Geometry check sheet. Reference: the model listing, model coordinates, mm. Face numbers are marked on the shaded views. A direction names the side the tool comes from. Give positions to 0.01 mm unless a question says otherwise; leave off trailing zeros. Order: outer loops, then holes, each group sorted by start corner. A loop starts at its lowest first (then second) coordinate and runs counter-clockwise, first axis right, second up. Notation, with made-up numbers: M -8,84.5 L -1,84.5 A20 cw -1,104.5 Z; hole C -16.5,51 d4. An arc over 180 degrees is marked long. Put each result on its own line as item: value. Start each with the question number.
Q1. Section check B-B on y = -164. Record the cut outline in (x, z), then the cut area to 3 significant figures.
Q2. Section check D-D on z = -3.25. Record the cut outline in (x, y), then the cut area to 3 significant figures.
Q3. Section check A-A on x = 0.75. Record the cut outline in (y, z), then the cut area to 3 significant figures.
Q4. Go/stop test with a flat-tipped pin: pin 1 (13.5 mm diameter, centred on y = -254, z = 0, fed in from +X). Record where the tip stops, or that it passes through.
Q5. Section check C-C on y = -54. Record the cut outline in (x, z).
Q6. Material ranges on L1, parallel to Y at x = 13.9, z = 0; L2, parallel to Z at x = 3.5, y = -181, recorded low to high.
Q7. Access from +Z, -Z, +X, -X, +Y, -Y to the whole of each face (thin tool, end or side, straight path). Record for the marked faces 1 and 2.
Q8. Mould release check, pull along Z, two halves, no side actions. Record for the marked faces 3, 4 and 5: +Z half, -Z half, draft (parallel to the pull), parting line (faces both ways), or undercut.
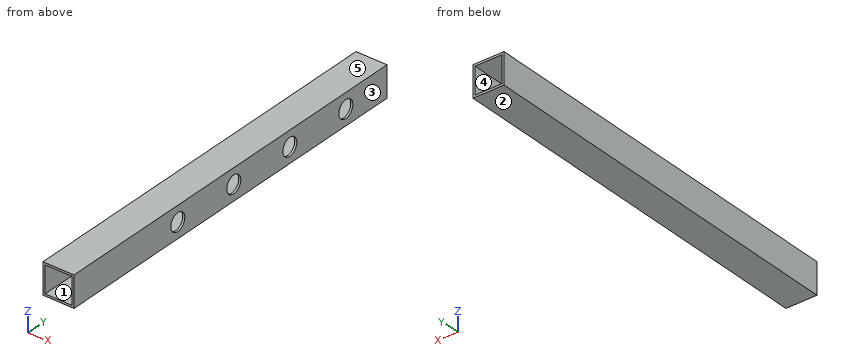
Autodesk Inventor part; units mm, degrees
ref_plane "YZ Plane" through (0, 0, 0) normal (1, 0, 0) x (0, 1, 0)
ref_plane "XZ Plane" through (0, 0, 0) normal (0, 1, 0) x (-1, 0, 0)
ref_plane "XY Plane" through (0, 0, 0) normal (0, 0, 1) x (1, 0, 0)
sketch "Sketch9" plane through (0, 0, 0) normal (0, 1, 0) x (-1, 0, 0)
  line L0 (15, 15) -> (-15, 15)
  line L1 (-15, 15) -> (-15, -15)
  line L2 (-15, -15) -> (15, -15)
  line L3 (15, -15) -> (15, 15)
  line L4 (15, 15) -> (-15, -15) construction
  line L5 (-15, 15) -> (15, -15) construction
  line L6 (-13, 13) -> (13, 13)
  line L7 (13, 13) -> (13, -13)
  line L8 (13, -13) -> (-13, -13)
  line L9 (-13, -13) -> (-13, 13)
  point P0 (0, 0)
  dimension "d172" = 30
  dimension "d173" = 30
  dimension "d174" = 2
extrude "Extrusion3" add sketch "Sketch9" against normal blind 380
sketch "Sketch10" plane through (0, 0, 0) normal (1, 0, 0) x (0, 1, 0)
  line L0 (0, 15) -> (0, -15) construction
  line L1 (0, 15) -> (-380, 15) construction
  line L2 (0, -15) -> (-380, -15) construction
  line L3 (-58.5, 8.5) -> (-41.5, 8.5)
  line L4 (-41.5, 8.5) -> (-41.5, -8.5)
  line L5 (-41.5, -8.5) -> (-58.5, -8.5)
  line L6 (-58.5, -8.5) -> (-58.5, 8.5)
  line L7 (-58.5, 8.5) -> (-41.5, -8.5) construction
  line L8 (-41.5, 8.5) -> (-58.5, -8.5) construction
  line L9 (0, 0) -> (30, 0)
  circle A0 centre (-50, 0) radius 8.5
  dimension "d177" = 17
  dimension "d178" = 17
  dimension "d181" = 30
  dimension "d182" = 80
extrude "Extrusion4" cut sketch "Sketch10" along normal through all contours A0
pattern_linear "Rectangular Pattern4" count 4 spacing 68 along (0, -1, 0) of "Extrusion4"
properties part number "PRS 1662 DrSysB way tube 4_D1200" material "Stainless Steel"
Results found:
1. outline: M -15,-15 L 15,-15 L 15,15 L -15,15 Z; hole M -13,-13 L 13,-13 L 13,13 L -13,13 Z
1. area: 224 mm^2
2. outline: M -15,-380 L -13,-380 L -13,0 L -15,0 Z; M 13,-380 L 15,-380 L 15,-261.85 L 13,-261.85 Z; M 13,-246.15 L 15,-246.15 L 15,-193.85 L 13,-193.85 Z; M 13,-178.15 L 15,-178.15 L 15,-125.85 L 13,-125.85 Z; M 13,-110.15 L 15,-110.15 L 15,-57.85 L 13,-57.85 Z; M 13,-42.15 L 15,-42.15 L 15,0 L 13,0 Z
2. area: 1,390 mm^2
3. outline: M -380,-15 L 0,-15 L 0,-13 L -380,-13 Z; M -380,13 L 0,13 L 0,15 L -380,15 Z
3. area: 1,520 mm^2
4. pin 1: stops at x = -13
5. outline: M -15,-15 L 15,-15 L 15,-7.5 L 13,-7.5 L 13,-13 L -13,-13 L -13,13 L 13,13 L 13,7.5 L 15,7.5 L 15,15 L -15,15 Z
6. L1: y = -380 to -262.5, -245.5 to -194.5, -177.5 to -126.5, -109.5 to -58.5, -41.5 to 0
6. L2: z = -15 to -13, 13 to 15
7. face 1: +Y, -Y
7. face 2: -Z, +X, -X, +Y, -Y
8. face 3: draft
8. face 4: undercut
8. face 5: +Z half
